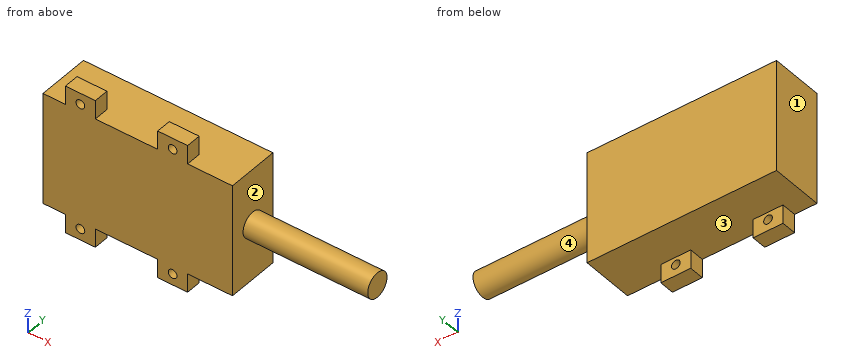
from build123d import *

# Parameters (mm, degrees)
SKETCH_1_W      = 76
SKETCH_1_H      = 45
EXTRUDE_1_DEPTH = 21
SKETCH_2_W      = 12
SKETCH_2_H      = 15
SKETCH_2_R      = 1.75
EXTRUDE_2_DEPTH = 6
SKETCH_3_R      = 5
EXTRUDE_3_DEPTH = 50


with BuildPart() as part:
    # 草图1 → 凸台-拉伸1 (new body)
    with BuildSketch(Plane(origin=(0, 0, 0), x_dir=(1, 0, 0), z_dir=(0, 1, 0))):
        Rectangle(SKETCH_1_W, SKETCH_1_H)
    extrude(amount=EXTRUDE_1_DEPTH)

    # 草图2 → 凸台-拉伸2 (add)
    with BuildSketch(Plane(origin=(0, 0, 0), x_dir=(1, 0, 0), z_dir=(0, 1, 0))):
        with Locations((-23, -22.5)):
            Rectangle(SKETCH_2_W, SKETCH_2_H)
        with Locations((-23, -25.5)):
            Circle(SKETCH_2_R, mode=Mode.SUBTRACT)
        with Locations((14, -22.5)):
            Rectangle(SKETCH_2_W, SKETCH_2_H)
        with Locations((14, -25.5)):
            Circle(SKETCH_2_R, mode=Mode.SUBTRACT)
        with Locations((14, 22.5)):
            Rectangle(SKETCH_2_W, SKETCH_2_H)
        with Locations((14, 25.5)):
            Circle(SKETCH_2_R, mode=Mode.SUBTRACT)
        with Locations((-23, 22.5)):
            Rectangle(SKETCH_2_W, SKETCH_2_H)
        with Locations((-23, 25.5)):
            Circle(SKETCH_2_R, mode=Mode.SUBTRACT)
    extrude(amount=EXTRUDE_2_DEPTH)

    # 草图3 → 凸台-拉伸3 (add)
    with BuildSketch(Plane(origin=(38, 0, 0), x_dir=(0, 0, -1), z_dir=(1, 0, 0))):
        with Locations((0, 10.5)):
            Circle(SKETCH_3_R)
    extrude(amount=EXTRUDE_3_DEPTH)


solid = part.part
Verification items for the finished model (mm, model axes). Face numbers are marked on the shaded views. Coordinates: 2 decimals unless noted, no trailing zeros. Order: outer loops, then holes, each group sorted by start corner. A loop starts at its lowest first (then second) coordinate and runs counter-clockwise, first axis right, second up. Notation, with made-up numbers: M 72,38 L 85,38 A17 ccw 85,54 Z; hole C -39.75,46.5 d11. An arc over 180 degrees is marked long. Write each question's results on one line, items separated by ' | '.
1) Gauge pin test, flat ends, axial feed: pin 1 Ø2 at (x, z) = (12.5, -25.5) entering from +Y; pin 2 Ø6.5 at (y, z) = (3.5, -28) entering from -X; pin 3 Ø5 at (y, z) = (2.5, -28) entering from +X. Record the tip position at first contact, or that the pin passes through.
Solved:
pin 1: stops at y = 6 | pin 2: stops at x = -29 | pin 3: stops at x = 20
2) Scan lines: line 1 along X through (y, z) = (3.2, -25.5); line 2 along Z through (x, y) = (14, 3.5); line 3 along Z through (x, y) = (31.5, 16.5). Record each from-to range of solid material in increasing order. Write a range as [from, to].
Solved:
line 1: x = [-29, -24.75], [-21.25, -17], [8, 12.25], [15.75, 20] | line 2: z = [-30, -27.25], [-23.75, 23.75], [27.25, 30] | line 3: z = [-22.5, 22.5]
3) Release check for a two-part mould opening along X. For the marked faces 1, 2, 3 and 4 record: pulls with the +X half, pulls with the -X half, needs draft (parallel to the pull), parting line crosses it, or undercut.
Solved:
face 1: pulls with the -X half | face 2: pulls with the +X half | face 3: undercut | face 4: needs draft
4) Section check D-D on y = 10.5. Record the cut outline in (x, z), plus the area to 3 significant figures.
Solved:
outline: M -38,-22.5 L 38,-22.5 L 38,-5 L 88,-5 L 88,5 L 38,5 L 38,22.5 L -38,22.5 Z | area: 3,920 mm²
5) Section check A-A on x = -23. Record the cut outline in (y, z).
Solved:
outline: M 0,-30 L 6,-30 L 6,-27.25 L 0,-27.25 Z; M 0,-23.75 L 6,-23.75 L 6,-22.5 L 21,-22.5 L 21,22.5 L 6,22.5 L 6,23.75 L 0,23.75 Z; M 0,27.25 L 6,27.25 L 6,30 L 0,30 Z
6) Section check B-B on z = -25.5. Record the cut outline in (x, y).
Solved:
outline: M -29,0 L -24.75,0 L -24.75,6 L -29,6 Z; M -21.25,0 L -17,0 L -17,6 L -21.25,6 Z; M 8,0 L 12.25,0 L 12.25,6 L 8,6 Z; M 15.75,0 L 20,0 L 20,6 L 15.75,6 Z
7) Section check C-C on y = 3.5. Record the cut outline in (x, z), plus the area to 3 significant figures.
Solved:
outline: M -38,-22.5 L -29,-22.5 L -29,-30 L -17,-30 L -17,-22.5 L 8,-22.5 L 8,-30 L 20,-30 L 20,-22.5 L 38,-22.5 L 38,22.5 L 20,22.5 L 20,30 L 8,30 L 8,22.5 L -17,22.5 L -17,30 L -29,30 L -29,22.5 L -38,22.5 Z; hole C -23,-25.5 d3.5; hole C -23,25.5 d3.5; hole C 14,-25.5 d3.5; hole C 14,25.5 d3.5 | area: 3,740 mm²
